Can you work these out from the model? Positions are in its coordinate system, mm. Face numbers are marked on the shaded views. A direction names the side the tool comes from. Round coordinates to 2 decimals unless told otherwise and drop trailing zeros. Loops run counter-clockwise (first coordinate to the right, second up) from the corner with the lowest first, then second, coordinate; pieces in that order, holes last. Notation, with made-up numbers: (40.5, -9.5) -> (72.5, -9.5) arc R14 cw to (72.5, 0.5) -> close; hole circle Ø8 at (13.25, 29.25). An arc over 180 degrees is marked (long way). Write each question's results on one line, items separated by ' | '.
from build123d import *

# Parameters (mm, degrees)
BOSS_EXTRUDE1_DEPTH = 32
CUT_EXTRUDE1_DEPTH  = 373.178248616
CUT_EXTRUDE2_DEPTH  = 373.178248616


with BuildPart() as part:
    # Sketch1 → Boss-Extrude1 (new body)
    with BuildSketch(Plane.XY):
        with BuildLine():
            Line((0, 0), (5.6712054, -40.352723193))
            ThreePointArc((5.6712054, -40.352723193), (75.270905948, -46.149494531), (136.31057695, -12.210145124))
            ThreePointArc((136.31057695, -12.210145124), (149.453776515, -3.178849861), (165.080769267, 0))
            Line((165.080769267, 0), (360, 0))
            Line((360, 0), (360, 40))
            Line((360, 40), (156.254224553, 40))
            ThreePointArc((156.254224553, 40), (131.195287612, 34.51650832), (110.716699745, 19.068322645))
            ThreePointArc((110.716699745, 19.068322645), (75.630846168, -4.623558298), (33.367064735, -7.092388553))
            Line((33.367064735, -7.092388553), (0, 0))
        make_face()
    extrude(amount=BOSS_EXTRUDE1_DEPTH)

    # Sketch3 → Cut-Extrude1 (cut, through all)
    with BuildSketch(Plane(origin=(0, 40, 0), x_dir=(1, 0, 0), z_dir=(0, 1, 0))):
        Polygon((155, -10), (156.254224553, -8.745775447), (156.254224553, 0), (0, 0), (0, -10), align=None)
        Polygon((156.254224553, -32), (156.254224553, -23.254224553), (155, -22), (0, -22), (0, -32), align=None)
        Polygon((156.254224553, -8.745775447), (165, 0), (156.254224553, 0), align=None)
        Polygon((165, -32), (156.254224553, -23.254224553), (156.254224553, -32), align=None)
    extrude(amount=-CUT_EXTRUDE1_DEPTH, mode=Mode.SUBTRACT)

    # Sketch4 → Cut-Extrude2 (cut, through all)
    with BuildSketch(Plane(origin=(0, 40, 0), x_dir=(1, 0, 0), z_dir=(0, 1, 0))):
        Polygon((0, -10), (155, -10), (154.5, -10.5), (14.318126641, -10.5), align=None)
        Polygon((0, -22), (14.318126641, -21.5), (154.5, -21.5), (155, -22), align=None)
    extrude(amount=-CUT_EXTRUDE2_DEPTH, mode=Mode.SUBTRACT)


solid = part.part
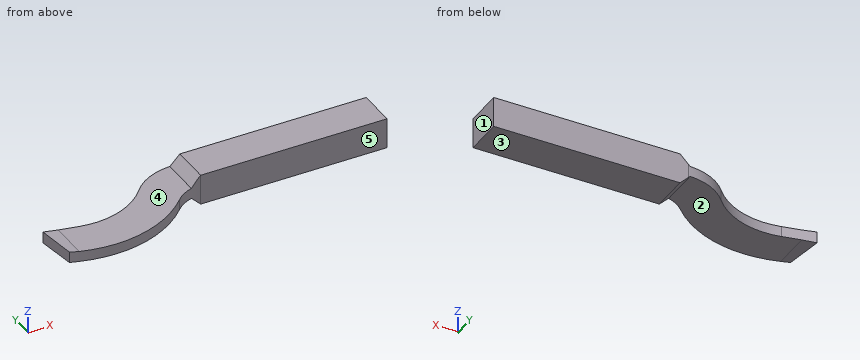
1. Will these pins go through, and if not, where does the flat tip stop? pin 1 (8 mm diameter, centred on x = 214, z = 23, fed in from -Y); pin 2 (5 mm diameter, centred on x = 55.5, z = 23, fed in from -Y); pin 3 (5 mm diameter, centred on x = 123.5, y = 22.5, fed in from -Z).
Final values:
pin 1: y = 0 | pin 2: y = -48.79 | pin 3: z = 10.5
2. If we section it at D-D (y = 6.5): List the corners of the cut face in (x, z) for me.
Final values:
outline: (97.11, 10.5) -> (154.5, 10.5) -> (165, 0) -> (360, 0) -> (360, 32) -> (165, 32) -> (154.5, 21.5) -> (97.11, 21.5) -> close
3. If we section it at A-A (z = 16): List the corners of the cut face in (x, y) for me.
Final values:
outline: (0, 0) -> (5.67, -40.35) arc R120 ccw to (136.31, -12.21) arc R40 cw to (165.08, 0) -> (360, 0) -> (360, 40) -> (156.25, 40) arc R60 ccw to (110.72, 19.07) arc R80 cw to (33.37, -7.09) -> close
4. If we section it at C-C (x = 199): List the corners of the cut face in (y, z) for me.
Final values:
outline: (0, 0) -> (40, 0) -> (40, 32) -> (0, 32) -> close
5. If we section it at B-B (y = 29.5): List the corners of the cut face in (x, z) for me.
Final values:
outline: (122.35, 10.5) -> (154.5, 10.5) -> (165, 0) -> (360, 0) -> (360, 32) -> (165, 32) -> (154.5, 21.5) -> (122.35, 21.5) -> close
6. On a 3-axis mill with a long thin cutter (end or side, diameter ignored), from which of +Z, -Z, +X, -X, +Y, -Y can I reach the whole of each face in a straight line? I mean the marked faces 1, 2, 3, 4 and 5. Say none if no direction works.
Final values:
face 1: +Z, -Z, +X, +Y, -Y | face 2: -Z, +Y, -Y | face 3: -Z, +X, -X, +Y, -Y | face 4: +Z, +Y, -Y | face 5: +Z, -Z, +X, -Y
7. Please list where these lines run through material, in increasing order: line 1 (Z direction, x = 72, y = -32); line 2 (Y direction, x = 280.5, z = 29); line 3 (Y direction, x = 49, z = 16.5). Write a range as from..to.
Final values:
line 1: 10.5..21.5 | line 2: 0..40 | line 3: -48.84..-8.83
